Geometry: final body of the model. Coordinates: model frame, mm. Face numbers are marked on the shaded views. A direction names the side the tool comes from. Give positions to 0.01 mm unless a question says otherwise; leave off trailing zeros. Write each loop counter-clockwise with the first axis right and the second up, starting at its lowest first coordinate (ties: lowest second). Pieces come first, ordered by that corner, then holes. Notation, with made-up numbers: (47.5, 31) -> (84.5, 31) arc R34 ccw to (84.5, 67) -> close; hole circle Ø3 at (-20.5, 81.5). An arc over 180 degrees is marked (long way). Answer in a Markdown table with one row per item. Add a question column.
Item 1: Access query for the marked faces 4, 5 and 6. Directions: +Z, -Z, +X, -X, +Y, -Y. A direction counts if a zero-diameter tool reaches every point of the face in a straight line with its end or side. Return the directions, or none.
Item 2: Section query B-B on z = 29. Output: boundary loops of the cut face in (x, y).
Item 3: Section query C-C on x = -449. Output: boundary loops of the cut face in (y, z).
Item 4: First-contact query: P1, Ø2, axis at x = -531, z = 35, coming from the +Y side; P2, Ø12, axis at y = 32.5, z = 34, coming from the +X side; P3, Ø10, axis at x = -262.5, z = 57.5, coming from the +Y side. Flat tips, straight axial feed; report the tip coordinate or a pass-through.
Item 5: Material intervals for probe 1 along X at (y, z) = (26, 58); probe 2 along X at (y, z) = (25.5, 50); probe 3 along X at (y, z) = (44, 39.5), sorted ascending. Write a range as from..to.
Item 6: Section query A-A on y = 12. Output: boundary loops of the cut face in (x, z).
Item 7: Draft query along X for the marked faces 1, 2 and 3. Return one class per face: +X half, -X half, draft (parallel to the pull), parting line (faces both ways), or undercut.
Item 8: Section query D-D on x = -249. Output: boundary loops of the cut face in (y, z).
```python
from build123d import *

# Parameters (mm, degrees)
BOSS_EXTRUDE1_DEPTH = 80


with BuildPart() as part:
    # Sketch1 → Boss-Extrude1 (new body)
    with BuildSketch(Plane.XY):
        with BuildLine():
            Line((0, 0), (-200, 0))
            ThreePointArc((-200, 0), (-300, 38.196601125), (-400, 0))
            Line((-400, 0), (-600, 0))
            Line((-600, 0), (-600, 30))
            Line((-600, 30), (-700, 30))
            Line((-700, 30), (-700, 55))
            Line((-700, 55), (-575, 55))
            Line((-575, 55), (-575, 25))
            Line((-575, 25), (-409.132167834, 25))
            ThreePointArc((-409.132167834, 25), (-300, 63.196601125), (-190.867832166, 25))
            Line((-190.867832166, 25), (0, 25))
            Line((0, 25), (0, 0))
        make_face()
    extrude(amount=BOSS_EXTRUDE1_DEPTH)


solid = part.part
```
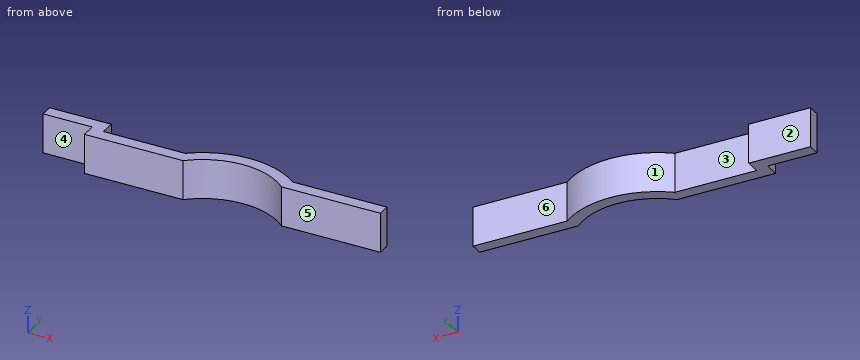
Findings below:
| question | item | result |
|---|---|---|
| 1 | face 4 | +Z, -Z, -X, -Y |
| 1 | face 5 | +Z, -Z, +X, -X, -Y |
| 1 | face 6 | +Z, -Z, +X, +Y |
| 2 | outline | (-700, 30) -> (-600, 30) -> (-600, 0) -> (-400, 0) arc R150 cw to (-200, 0) -> (0, 0) -> (0, 25) -> (-190.87, 25) arc R175 ccw to (-409.13, 25) -> (-575, 25) -> (-575, 55) -> (-700, 55) -> close |
| 3 | outline | (0, 0) -> (25, 0) -> (25, 80) -> (0, 80) -> close |
| 4 | P1 | stops at y = 25 |
| 4 | P2 | stops at x = -192.78 |
| 4 | P3 | stops at y = 60.15 |
| 5 | probe 1 | x = -600..-575, -407.87..-359.25, -240.75..-192.13 |
| 5 | probe 2 | x = -600..-575, -408.5..-360.4, -239.6..-191.5 |
| 5 | probe 3 | x = -700..-575, -379.69..-220.31 |
| 6 | outline | (-600, 0) -> (-384.69, 0) -> (-384.69, 80) -> (-600, 80) -> close; (-215.31, 0) -> (0, 0) -> (0, 80) -> (-215.31, 80) -> close |
| 7 | face 1 | undercut |
| 7 | face 2 | draft |
| 7 | face 3 | undercut |
| 8 | outline | (29.26, 0) -> (55.6, 0) -> (55.6, 80) -> (29.26, 80) -> close |
